Source: CAD feature listing. Evaluate the final solid. Frame: model axes, mm. Face numbers are marked on the shaded views. A direction names the side the tool comes from. Give positions to 0.01 mm unless a question says otherwise; leave off trailing zeros. Order: outer loops, then holes, each group sorted by start corner. A loop starts at its lowest first (then second) coordinate and runs counter-clockwise, first axis right, second up. Notation, with made-up numbers: M 9,-16 L 48,-16 A7 ccw 48,-7 Z; hole C 36.5,31.5 d1. An arc over 180 degrees is marked long. Use CSV: the item, a comma, the result in double quotes. Start each with the question number.
1. Pin query (flat end, axial travel): P1, Ø1.5, axis at x = -1.5, y = 9, coming from the -Z side; P2, Ø0.5, axis at x = 3.5, y = -8, coming from the +Z side; P3, Ø4, axis at x = 2, y = 6, coming from the +Z side; P4, Ø8, axis at y = 8, z = 19.5, coming from the +X side. Return the tip coordinate at first contact, or that it passes through.
2. Reachability of the marked faces 1, 2 and 3 from +Z, -Z, +X, -X, +Y, -Y: full face, straight path, thin tool, end or side. Return the list, or none.
3. Mould query, pull axis Y, two halves, no side actions, for the marked faces 4, 5, 6 and 7. Classes: released by +Y, released by -Y, zero draft, split by the parting line, or undercut.
4. Section query D-D, the plane z = 16.5. Return the cut outline in (x, y).
5. Section query B-B, the plane z = 42. Return the cut outline in (x, y), plus the area to 3 significant figures.
6. Section query A-A, the plane y = 9.5. Return the cut outline in (x, z).
7. Section query C-C, the plane y = -3.25. Return the cut outline in (x, z).
8. Line query: line 1 along Y through (x, z) = (-5.5, 8.5); line 2 along Z through (x, y) = (4.5, -6); line 3 along Y through (x, z) = (5.5, 18). Output: solid intervals per line, ascending. Write a range as [from, to].
from build123d import *

# Parameters (mm, degrees)
F0_W      = 15
F0_H      = 8.5
F1_DEPTH  = 15
F2_W      = 15
F2_H      = 6.5
F3_DEPTH  = 1
F4_W      = 6.5
F4_H      = 14
F5_DEPTH  = 1
F6_W      = 14
F6_H      = 6.5
F7_DEPTH  = 1
F8_W      = 6.5
F8_H      = 13
F9_DEPTH  = 1
F10_W     = 5
F10_H     = 1
F11_DEPTH = 5
F12_W     = 9
F12_H     = 9
F13_DEPTH = 2
F17_DEPTH = 25


with BuildPart() as f1:
    # F0 (on Top) → F1 (new body)
    with BuildSketch(Plane.XY):
        with Locations((0, -4.25)):
            Rectangle(F0_W, F0_H)
    extrude(amount=F1_DEPTH)

    # F2 (on face) → F3 (cut)
    with BuildSketch(Plane.XY.offset(15)):
        with Locations((0, -4.25)):
            Rectangle(F2_W, F2_H)
    extrude(amount=-F3_DEPTH, mode=Mode.SUBTRACT)

    # F4 (on face) → F5 (cut)
    with BuildSketch(Plane.YZ.offset(7.5)):
        with Locations((-4.25, 7)):
            Rectangle(F4_W, F4_H)
    extrude(amount=-F5_DEPTH, mode=Mode.SUBTRACT)

    # F6 (on face) → F7 (cut)
    with BuildSketch(Plane(origin=(0, 0, 0), x_dir=(1, 0, 0), z_dir=(0, 0, -1))):
        with Locations((-0.5, 4.25)):
            Rectangle(F6_W, F6_H)
    extrude(amount=-F7_DEPTH, mode=Mode.SUBTRACT)

    # F8 (on face) → F9 (cut)
    with BuildSketch(Plane(origin=(-7.5, 0, 0), x_dir=(0, -1, 0), z_dir=(-1, 0, 0))):
        with Locations((4.25, 7.5)):
            Rectangle(F8_W, F8_H)
    extrude(amount=-F9_DEPTH, mode=Mode.SUBTRACT)

    # F10 (on face) → F11 (join)
    with BuildSketch(Plane.XY.offset(15)):
        with Locations((5, -8)):
            Rectangle(F10_W, F10_H)
    extrude(amount=F11_DEPTH)

    # F12 (on face) → F13 (join)
    with BuildSketch(Plane(origin=(0, 0, 0), x_dir=(-1, 0, 0), z_dir=(0, 1, 0))):
        with Locations((0, 7.5)):
            Rectangle(F12_W, F12_H)
    extrude(amount=F13_DEPTH)

    # F14 (on Right) → F15 (revolve)
    with BuildSketch(Plane.YZ):
        with BuildLine():
            ThreePointArc((4.196024, 11.486574), (3.124753, 11.857664), (2, 12))
            Line((2, 12), (2, 7.5))
            Line((2, 7.5), (12, 7.5))
            Line((12, 7.5), (12, 12.5))
            Line((12, 12.5), (8.965219, 12.5))
            ThreePointArc((8.965219, 12.5), (6.750409, 11.194264), (4.196024, 11.486574))
        make_face()
    revolve(axis=Axis((0, 7, 7.5), (0, 1, 0)))

    # F16 (on face) → F17 (join)
    with BuildSketch(Plane.XY.offset(20)):
        with BuildLine():
            Line((4, -8.5), (6, -8.5))
            ThreePointArc((6, -8.5), (5.707107, -7.792893), (5, -7.5))
            ThreePointArc((5, -7.5), (4.292893, -7.792893), (4, -8.5))
        make_face()
        with BuildLine():
            ThreePointArc((4, -8.5), (5, -9.5), (6, -8.5))
            Line((6, -8.5), (4, -8.5))
        make_face()
    extrude(amount=F17_DEPTH)


solid = f1.part
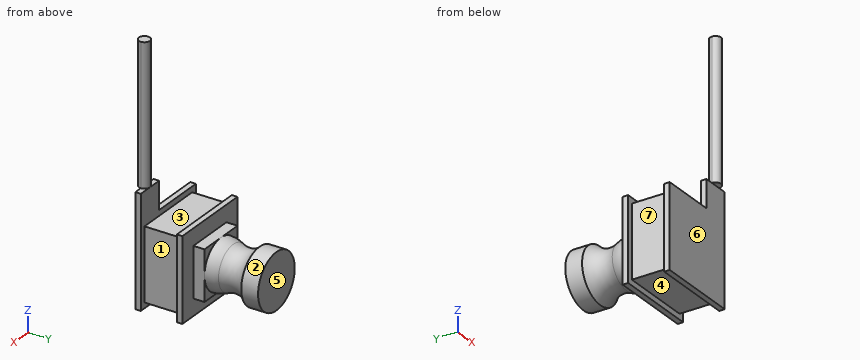
Result set:
1,P1,"z = 2.56"
1,P2,"z = 20"
1,P3,"z = 11.42"
1,P4,"through"
2,face 1,"+Z, -Z, +X"
2,face 2,"+Y"
2,face 3,"+Z, +X, -X"
3,face 4,"undercut"
3,face 5,"released by +Y"
3,face 6,"released by -Y"
3,face 7,"undercut"
4,outline,"M 2.5,-8.5 L 7.5,-8.5 L 7.5,-7.5 L 2.5,-7.5 Z"
5,outline,"C 5,-8.5 d2"
5,area,"3.14 mm2"
6,outline,"C 0,7.5 d10"
7,outline,"M -6.5,1 L 6.5,1 L 6.5,14 L -6.5,14 Z"
8,line 1,"[-8.5, 0]"
8,line 2,"[1, 14]"
8,line 3,"[-8.5, -7.5]"
